Build history of the part. All positions in model axes, mm. Coordinates: 2 decimals unless noted, no trailing zeros. Order: outer loops, then holes, each group sorted by start corner. A loop starts at its lowest first (then second) coordinate and runs counter-clockwise, first axis right, second up. Notation, with made-up numbers: (65.25, 85.5) - (108.25, 85.5) arc R14 ccw to (108.25, 105.5) - close; hole circle Ø2 at (79.5, -13). An arc over 180 degrees is marked (long way). One line per item, written item: value.
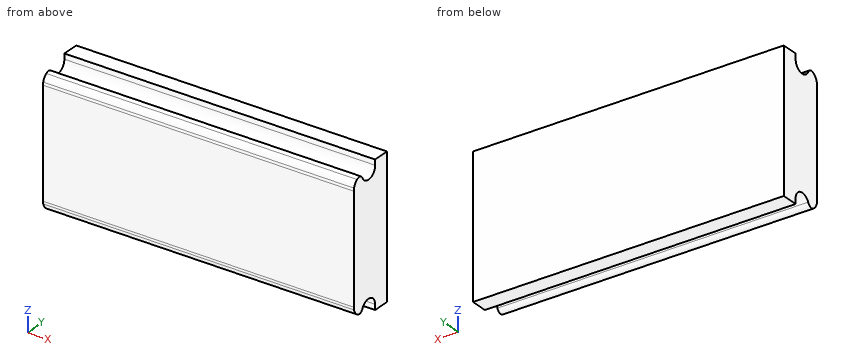
from build123d import *

# Parameters (mm, degrees)
BOSS_EXTRUDE1_DEPTH = 73.824999924


with BuildPart() as part:
    # Sketch1 → Boss-Extrude1 (new body)
    with BuildSketch(Plane(origin=(0, 0, 0), x_dir=(0, 0, -1), z_dir=(1, 0, 0))):
        with BuildLine():
            Line((-15.345833333, 15.875), (-16.615833333, 15.875))
            Line((-16.615833333, 15.875), (-16.615833333, 11.90625))
            Line((-16.615833333, 11.90625), (-15.345833333, 11.90625))
            ThreePointArc((-15.345833333, 11.90625), (-13.186497119, 10.205674607), (-14.333561104, 7.707888834))
            add(Edge.make_bspline(
                [(-14.893216846, 5.855285409), (-15.624772824, 7.07621566), (-14.333561104, 7.707888834)],
                knots=[0, 0, 0, 1, 1, 1], degree=2))
            ThreePointArc((-14.893216846, 5.855285409), (-14.258115568, 5.218639085), (-13.44097879, 4.843193137))
            ThreePointArc((-13.44097879, 4.843193137), (-13.125958752, 4.782754037), (-12.805833333, 4.7625))
            Line((-12.805833333, 4.7625), (12.805833333, 4.7625))
            ThreePointArc((12.805833333, 4.7625), (13.125958752, 4.782754037), (13.44097879, 4.843193137))
            ThreePointArc((13.44097879, 4.843193137), (14.258115568, 5.218639085), (14.893216846, 5.855285409))
            add(Edge.make_bspline(
                [(14.893216846, 5.855285409), (15.624772824, 7.07621566), (14.333561104, 7.707888834)],
                knots=[0, 0, 0, 1, 1, 1], degree=2))
            ThreePointArc((14.333561104, 7.707888834), (13.186497119, 10.205674607), (15.345833333, 11.90625))
            Line((15.345833333, 11.90625), (16.615833333, 11.90625))
            Line((16.615833333, 11.90625), (16.615833333, 15.875))
            Line((16.615833333, 15.875), (15.345833333, 15.875))
            Line((15.345833333, 15.875), (-15.345833333, 15.875))
        make_face()
    extrude(amount=BOSS_EXTRUDE1_DEPTH)


solid = part.part
1. Band-saw the part on A-A, the plane y = 8.75. Give the cut face in (x, z) (3 decimals), and give its area (3 significant figures).
Values found:
outline: (0, -13.331) - (73.825, -13.331) - (73.825, 13.331) - (0, 13.331) - close
area: 1,970 mm2
2. Probe line 1 along Y through (x, z) = (3.5, 13) (3 decimals); line 2 along Y through (x, z) = (47.5, -14.5) (3 decimals); line 3 along Z through (x, y) = (50.5, 9.5). List the from-to ranges inside material, lowest first.
Values found:
line 1: y = 4.77 to 15.875
line 2: y = 5.41 to 7.619, 11.739 to 15.875
line 3: z = -13.13 to 13.13
3. Flat gauge pins, fed straight in: P1, Ø1, axis at x = 34.5, z = 16, coming from the -Y side; P2, Ø1.4, axis at x = 18.5, z = -15.5, coming from the -Y side; P3, Ø3, axis at x = 19, y = 10, coming from the +Z side. Where does each tip first touch, or does it go through?
Values found:
P1: stops at y = 11.91
P2: stops at y = 5.73
P3: stops at z = 14.07
